For this review, take the finished solid that the model builds, in its own axes (mm). A direction names the side the tool comes from. Coordinates: 2 decimals unless noted, no trailing zeros. Write each loop counter-clockwise with the first axis right and the second up, starting at its lowest first coordinate (ties: lowest second). Pieces come first, ordered by that corner, then holes. Notation, with made-up numbers: M 52.25,62.5 L 70.25,62.5 A6 cw 70.25,71.5 Z; hole C -37,79.25 d5. An arc over 180 degrees is marked long. Return JSON: item names as keys, results as strings.
```python
from build123d import *

# Parameters (mm, degrees)
SKETCH2_R          = 3.3
CUT_EXTRUDE1_DEPTH = 41
SKETCH3_W          = 12
SKETCH3_H          = 2
CUT_EXTRUDE2_DEPTH = 47


with BuildPart() as part:
    # Sketch1 → Revolve1 (revolve)
    with BuildSketch(Plane(origin=(0, 0, 0), x_dir=(1, 0, 0), z_dir=(0, 1, 0))):
        Polygon((0, 23), (46, 23), (46, 33), (16, 33), (16, 47), (6, 47), (6, 28), (0, 28), align=None)
    revolve(axis=Axis((-31.159383033, 0, 0), (1, 0, 0)))

    # Sketch2 → Cut-Extrude1 (cut, through all)
    with BuildSketch(Plane.ZY.offset(-6)):
        with Locations((0, 40)):
            Circle(SKETCH2_R)
        with Locations((34.641016151, 20)):
            Circle(SKETCH2_R)
        with Locations((34.641016151, -20)):
            Circle(SKETCH2_R)
        with Locations((0, -40)):
            Circle(SKETCH2_R)
        with Locations((-34.641016151, -20)):
            Circle(SKETCH2_R)
        with Locations((-34.641016151, 20)):
            Circle(SKETCH2_R)
    extrude(amount=-CUT_EXTRUDE1_DEPTH, mode=Mode.SUBTRACT)

    # Sketch3 → Cut-Extrude2 (cut, through all)
    with BuildSketch(Plane.ZY):
        with Locations((0, -23.203603311)):
            Rectangle(SKETCH3_W, SKETCH3_H)
    extrude(amount=-CUT_EXTRUDE2_DEPTH, mode=Mode.SUBTRACT)


solid = part.part
```
1. Draft analysis for pull direction Y (two halves, no side actions). For faces 5 (the face through (10.93, 18.74, -31.59)), 6 (the face through (2.958, -10.724, -25.865)), 7 (the face through (10.93, -21.26, -31.59)), 8 (the face through (46, 22.5, 6.9)), state which applies: +Y half, -Y half, draft (parallel to the pull), parting line (faces both ways), or undercut.
Checks:
{"face 5": "undercut", "face 6": "parting line", "face 7": "undercut", "face 8": "draft"}
2. For faces 1 (the face through (23, -24.204, 0)), 2 (the face through (6, -20, -20)), 3 (the face through (16, -10, -32)), 4 (the face through (0, -21, -10)), list the 3-axis set-ups (+Z, -Z, +X, -X, +Y, -Y) from which the entire face can be reached by the end or side of a thin tool; tool diameter is ignored.
Checks:
{"face 1": "+X, -X", "face 2": "-X", "face 3": "+X", "face 4": "+Z, -Z, -X, +Y, -Y"}
3. We need section C-C (x = 10). State the section outline as (y, z) points, plus the area to 4 significant figures.
Checks:
{"outline": "C 0,0 d94; hole C -40,0 d6.6; hole M -24.2,-6 L -22.2,-6 A23 ccw long -22.2,6 L -24.2,6 Z; hole C -20,-34.64 d6.6; hole C -20,34.64 d6.6; hole C 20,-34.64 d6.6; hole C 20,34.64 d6.6; hole C 40,0 d6.6", "area": "5,055 mm2"}
4. Wall thickness on L1, parallel to Y at x = 17, z = 0; L2, parallel to X at y = 24.5, z = -33; L3, parallel to X at y = 30.5, z = -10: over which ranges is each line inside the solid? List them lowest first. Write a range as from..to.
Checks:
{"L1": "-33..-24.2, 23..33", "L2": "6..16", "L3": "6..46"}
5. We need section A-A (y = 0). State the section outline as (x, z) points, plus the area to 3 significant figures.
Checks:
{"outline": "M 0,-28 L 6,-28 L 6,-47 L 16,-47 L 16,-33 L 46,-33 L 46,-23 L 0,-23 Z; M 0,23 L 46,23 L 46,33 L 16,33 L 16,47 L 6,47 L 6,28 L 0,28 Z", "area": "1,140 mm2"}
6. Clearance check with flat-ended pins moving along their axes: pin 1 Ø0.6 at (x, y) = (34.5, -23) entering from -Z; pin 2 Ø8 at (x, y) = (35.5, 37.5) entering from -Z; pin 3 Ø1.6 at (x, y) = (12, -23.5) entering from +Z; pin 4 Ø1 at (y, z) = (31, -31.5) entering from +X. State where each tip first meets the part, or that it passes through.
Checks:
{"pin 1": "z = -23.95", "pin 2": "through", "pin 3": "z = 41.15", "pin 4": "x = 16"}
7. We need section D-D (x = 24.5). State the section outline as (y, z) points, plus the area to 3 significant figures.
Checks:
{"outline": "C 0,0 d66; hole M -24.2,-6 L -22.2,-6 A23 ccw long -22.2,6 L -24.2,6 Z", "area": "1,740 mm2"}
8. We need section B-B (z = 0). State the section outline as (x, y) points, plus the area to 3 significant figures.
Checks:
{"outline": "M 0,-28 L 6,-28 L 6,-36.7 L 16,-36.7 L 16,-33 L 46,-33 L 46,-24.2 L 0,-24.2 Z; M 0,23 L 46,23 L 46,33 L 16,33 L 16,36.7 L 6,36.7 L 6,28 L 0,28 Z; M 6,-47 L 16,-47 L 16,-43.3 L 6,-43.3 Z; M 6,43.3 L 16,43.3 L 16,47 L 6,47 Z", "area": "953 mm2"}
